Input: part model. Units: mm. Frame: model coordinates. A direction names the side the tool comes from. Coordinates: 2 decimals unless noted, no trailing zeros. Order: outer loops, then holes, each group sorted by start corner. A loop starts at its lowest first (then second) coordinate and runs counter-clockwise, first axis right, second up.
from build123d import *

# Parameters (mm, degrees)
F0_W     = 76.2
F0_H     = 127
F0_R     = 12.7
F1_DEPTH = 91.44
F2_W     = 30.48
F2_H     = 50.8
F3_DEPTH = 143.256
F4_T     = -2.54
F5_DEPTH = 20.32


with BuildPart() as f1:
    # F0 (on Top) → F1 (new body)
    with BuildSketch(Plane.XY):
        with Locations((-16.1199760675, 63.5)):
            Rectangle(F0_W, F0_H)
        with Locations((-16.1199760675, 63.5)):
            Circle(F0_R, mode=Mode.SUBTRACT)
    extrude(amount=F1_DEPTH)

    # F2 (on face) → F3 (cut)
    with BuildSketch(Plane(origin=(0, 127, 0), x_dir=(-1, 0, 0), z_dir=(0, 1, 0))):
        with Locations((16.1199760675, 46.99)):
            Rectangle(F2_W, F2_H)
    extrude(amount=-F3_DEPTH, mode=Mode.SUBTRACT)

    # F4
    f4_openings = [f1.faces().sort_by_distance(p)[0] for p in [
        (21.980024, 63.5, 45.72),
        (-54.219976, 63.5, 45.72),
    ]]
    offset(amount=F4_T, openings=f4_openings, kind=Kind.INTERSECTION)

    # F5 (add): a face of the model
    f5_faces = [f1.faces().sort_by_distance(p)[0] for p in [
        (1.6600239325, 63.5, 46.99),
    ]]
    extrude(f5_faces, amount=F5_DEPTH)


solid = f1.part
Item 1: Cut plane A-A on y = 36.5. Return loops of the section in (x, z).
Response values:
outline: (-54.22, 0) - (21.98, 0) - (21.98, 2.54) - (-54.22, 2.54) - close; (-54.22, 88.9) - (21.98, 88.9) - (21.98, 91.44) - (-54.22, 91.44) - close; (-33.9, 19.05) - (21.98, 19.05) - (21.98, 74.93) - (-33.9, 74.93) - close; hole (-31.36, 21.59) - (-0.88, 21.59) - (-0.88, 72.39) - (-31.36, 72.39) - close
Item 2: Cut plane B-B on x = -20. Count the separate pieces of the cut face and the enclosed holes in it, then the cut area to 3 significant figures.
Response values:
separate pieces: 4
enclosed holes: 4
area: 1,360 mm2
Item 3: Draft query along Y for faces 1 (the face through (21.98, 64, 45)), 2 (the face through (-34, 0, 45)), 3 (the face through (-42, 124.46, 36)). Return one class per face: pulls with the +Y half, pulls with the -Y half, needs draft (parallel to the pull), parting line crosses it, or undercut.
Response values:
face 1: needs draft
face 2: pulls with the -Y half
face 3: undercut
Item 4: Access query for faces 4 (the face through (-29, 64, 21.59)), 5 (the face through (-25, 78, 2.54)), 6 (the face through (-17.773, 76.092, 10.644)), 7 (the face through (-42, 2.54, 36)), 8 (the face through (-54.22, 2, 46)). Directions: +Z, -Z, +X, -X, +Y, -Y. A direction counts if a zero-diameter tool reaches every point of the face in a straight line with its end or side. Return the directions, or none.
Response values:
face 4: +Y, -Y
face 5: none
face 6: +Z, -Z
face 7: -X
face 8: +Z, -Z, -X, +Y, -Y
Item 5: Cut plane C-C on z = 48. Return loops of the section in (x, y), then the cut area to 3 significant figures.
Response values:
outline: (-54.22, 0) - (-31.36, 0) - (-31.36, 127) - (-54.22, 127) - (-54.22, 124.46) - (-33.9, 124.46) - (-33.9, 2.54) - (-54.22, 2.54) - close; (-0.88, 0) - (21.98, 0) - (21.98, 127) - (-0.88, 127) - close
area: 3,330 mm2
Item 6: Ray query, probe 1 along Z at (x, y) = (-6.5, 122); probe 2 along Z at (x, y) = (16, 76); probe 3 along Z at (x, y) = (-7, 75.5). Return the intervals inside material, ascending.
Response values:
probe 1: z = 0 to 2.54, 19.05 to 21.59, 72.39 to 74.93, 88.9 to 91.44
probe 2: z = 0 to 2.54, 19.05 to 74.93, 88.9 to 91.44
probe 3: z = 0 to 21.59, 72.39 to 91.44
Item 7: Pin query (flat end, axial travel): pin 1 Ø4 at (y, z) = (75, 80) entering from -X; pin 2 Ø24.5 at (x, y) = (-23, 93.5) entering from -Z; pin 3 Ø15 at (x, y) = (-16.12, 63.5) entering from -Z; pin 4 Ø12 at (y, z) = (50, 70.5) entering from -X. Return the tip coordinate at first contact, or that it passes through.
Response values:
pin 1: stops at x = -28.04
pin 2: stops at z = 0
pin 3: passes through
pin 4: stops at x = -33.9
